Input: part model. Units: mm. Frame: model coordinates. A direction names the side the tool comes from. Coordinates: 2 decimals unless noted, no trailing zeros. Write each loop counter-clockwise with the first axis right and the second up, starting at its lowest first coordinate (ties: lowest second). Pieces come first, ordered by that corner, then holes. Notation, with made-up numbers: (9.5, -8.75) - (17.5, -8.75) arc R21 ccw to (17.5, -1.75) - close; hole circle Ø1 at (66.5, -2.5). An arc over 180 degrees is marked (long way). One line per question, with ' | ' between items. Start each with the question number.
1) Section query A-A on y = 11.5. Return loops of the section in (x, z).
2) Section query B-B on x = 0. Return loops of the section in (y, z).
3) Section query D-D on z = 3.2. Return loops of the section in (x, y), and give its area (3 significant figures).
4) Draft query along X for faces 3 (the flat face through (5, -34, 4)), 4 (the cylindrical face through (0, -88, 2)), 5 (the flat face through (21.982, -23, 2)), 6 (the cylindrical face through (-15.76, 9.517, 1.972)). Return one class per face: released by +X, released by -X, zero draft, split by the parting line, or undercut.
5) First-contact query: P1, Ø1, axis at x = 15.5, z = 3.5, coming from the -Y side; P2, Ø1.5, axis at y = -6, z = 1.5, coming from the +X side; P3, Ø1.6, axis at x = -0.5, z = 3, coming from the -Y side. Flat tips, straight axial feed; report the tip coordinate or a pass-through.
6) Reachability of faces 1 (the flat face through (0, -71.25, 3)), 2 (the cylindrical face through (5.77, -14.42, 2.03)) from +Z, -Z, +X, -X, +Y, -Y: full face, straight path, thin tool, end or side. Return the list, or none.
7) Section query C-C on y = -78. Return loops of the section in (x, z).
8) Line query: line 1 (Y direction, x = 15, z = 3.6); line 2 (Y direction, x = -1, z = 1.25); line 3 (X direction, y = -21.5, z = 1.4). Output: solid intervals per line, ascending.
Autodesk Inventor part; units mm, degrees
ref_plane "YZ Plane" through (0, 0, 0) normal (1, 0, 0) x (0, 1, 0)
ref_plane "XZ Plane" through (0, 0, 0) normal (0, 1, 0) x (-1, 0, 0)
ref_plane "XY Plane" through (0, 0, 0) normal (0, 0, 1) x (1, 0, 0)
sketch "Sketch1" plane through (0, 0, 0) normal (0, 0, 1) x (1, 0, 0)
  line L0 (-22, 18.0955) -> (21.9822, 18.0955)
  line L1 (21.9822, 18.0955) -> (21.9822, -66)
  line L2 (-22, -66) -> (-22, 18.0955)
  arc A0 (-22, -65.3741) -> (21.9822, -65.3741) centre (-0.0089, -66) ccw
  point P0 (0, 0)
  dimension "d22" = 44
extrude "Base" add sketch "Sketch1" along normal blind 4
sketch "Sketch2" plane through (0, 0, 0) normal (0, 0, 1) x (1, 0, 0)
  circle A0 centre (-15.5, 11.5) radius 2
  circle A1 centre (15.5, 11.5) radius 2
  circle A2 centre (-15.5, -20.5) radius 2
  circle A3 centre (15.5, -20.5) radius 2
  point P0 (0, 0)
extrude "Mounting Holes" cut sketch "Sketch2" along normal blind 4
sketch "Sketch3" plane through (0, 0, 0) normal (0, 0, 1) x (1, 0, 0)
  circle A0 centre (0, -78) radius 2.5
  point P0 (0, 0)
  dimension "d24" = 5
extrude "Pivot Hole" cut sketch "Sketch3" along normal blind 4
ref_plane "Work Plane2" through (0, -60, 0) normal (0, 1, 0) x (-1, 0, 0)
sketch "Sketch4" plane through (0, -60, 0) normal (0, 1, 0) x (-1, 0, 0)
  circle A0 centre (0, 4) radius 2
  point P0 (0, 0)
  dimension "d14" = 4
extrude "Support Ridge" cut sketch "Sketch4" along normal blind 31.75 and the other way blind 11.25
sketch "Sketch5" plane through (0, 0, 4) normal (0, 0, 1) x (1, 0, 0)
  circle A0 centre (0, -3.3333) radius 12.5
  point P0 (0, 0)
  dimension "d19" = 25
extrude "Shaft Hole" cut sketch "Sketch5" against normal blind 4
properties part number "DispenserBrace3gallon"
Answer key:
1) outline: (-22, 0) - (-17.5, 0) - (-17.5, 4) - (-22, 4) - close; (-13.5, 0) - (13.5, 0) - (13.5, 4) - (-13.5, 4) - close; (17.5, 0) - (21.98, 0) - (21.98, 4) - (17.5, 4) - close
2) outline: (-88, 0) - (-80.5, 0) - (-80.5, 4) - (-88, 4) - close; (-75.5, 0) - (-15.83, 0) - (-15.83, 4) - (-28.25, 4) - (-28.25, 2) - (-71.25, 2) - (-71.25, 4) - (-75.5, 4) - close; (9.17, 0) - (18.1, 0) - (18.1, 4) - (9.17, 4) - close
3) outline: (-22, -65.37) arc R22 ccw (long way) to (21.98, -65.37) - (21.98, 18.1) - (-22, 18.1) - close; hole circle Ø4 at (-15.5, -20.5); hole circle Ø4 at (-15.5, 11.5); hole circle Ø25 at (0, -3.33); hole circle Ø5 at (0, -78); hole (-1.83, -71.25) - (1.83, -71.25) - (1.83, -28.25) - (-1.83, -28.25) - close; hole circle Ø4 at (15.5, -20.5); hole circle Ø4 at (15.5, 11.5) | area: 3,740 mm²
4) face 3: zero draft | face 4: split by the parting line | face 5: released by +X | face 6: undercut
5) P1: y = -82.09 | P2: x = 21.98 | P3: y = -88
6) face 1: +Z | face 2: +Z, -Z
7) outline: (-18.45, 0) - (-2.5, 0) - (-2.5, 4) - (-18.45, 4) - close; (2.5, 0) - (18.43, 0) - (18.43, 4) - (2.5, 4) - close
8) line 1: -82.09 to -22.44, -18.56 to 9.56, 13.44 to 18.1 | line 2: -87.98 to -80.29, -75.71 to -15.79, 9.13 to 18.1 | line 3: -22 to -17.23, -13.77 to 13.77, 17.23 to 21.98
